Model file for the job. Use its own axes, mm. A direction names the side the tool comes from. Round coordinates to 2 decimals unless told otherwise and drop trailing zeros. Order: outer loops, then holes, each group sorted by start corner. A loop starts at its lowest first (then second) coordinate and runs counter-clockwise, first axis right, second up. Notation, with made-up numbers: (-12, -6) -> (41, -6) arc R26 cw to (41, 16) -> close; hole circle Ø6 at (-31.5, 8). An arc over 180 degrees is marked (long way). Put each result on its own line as item: value. Start each with the question number.
Q1. Pull direction Y, two halves, no side cores. Call faces 4 (the face through (-1.46, -6.59, 40.6)), 5 (the face through (7.62, -3.16, 41.34)), 6 (the face through (-5.75, -5.27, 0.79)), 7 (the face through (-7, 0, 65)): released by +Y, released by -Y, zero draft, split by the parting line, or undercut.
Q2. Cut at A-A, the plane y = 0. List the corners of the cut face in (x, z).
Q3. Cut at D-D, the plane z = 11. List the corners of the cut face in (x, y).
Q4. Cut at C-C, the plane z = 58.5. List the corners of the cut face in (x, y), and give its area (3 significant figures).
Q5. Probe L1, parallel to Y at x = 0, z = 0.85; L2, parallel to Z at x = -6.25, y = 3.75; L3, parallel to Y at x = 0.25, z = 16.5. List the from-to ranges inside material, lowest first.
Q6. Flat gauge pins, fed straight in: P1, Ø6, axis at x = 1.5, z = 41.5, coming from the +Y side; P2, Ø2, axis at x = 4.5, z = 50, coming from the +Y side; P3, Ø4, axis at y = 4, z = 52, coming from the -X side. Where does each tip first touch, or does it go through?
Q7. 3-axis set-ups, long thin cutter, end or side, ignore diameter. For faces 1 (the face through (0, 0, 1.6)), 2 (the face through (-1.73, -7.81, 9.21)), 3 (the face through (-3, 8, 17)): which of +Z, -Z, +X, -X, +Y, -Y reach the whole face in a straight line?
from build123d import *

# Parameters (mm, degrees)
F0_R     = 9.5
F1_DEPTH = 65
F2_R     = 0.2
F3_R     = 9.5
F3_R_2   = 8.25
F4_DEPTH = 48
F5_R     = 7.8
F6_DEPTH = 1.6
F7_T     = -1.5


with BuildPart() as f1:
    # F0 (on Top) → F1 (new body)
    with BuildSketch(Plane.XY):
        Circle(F0_R)
    extrude(amount=F1_DEPTH)

    # F2
    f2_edges = [f1.edges().sort_by_distance(p)[0] for p in [
        (-9.5, 0, 0),
    ]]
    fillet(f2_edges, radius=F2_R)

    # F3 (on face) → F4 (cut)
    with BuildSketch(Plane.XY.offset(65)):
        Circle(F3_R)
        Circle(F3_R_2, mode=Mode.SUBTRACT)
    extrude(amount=-F4_DEPTH, mode=Mode.SUBTRACT)

    # F5 (on face) → F6 (cut)
    with BuildSketch(Plane(origin=(0, 0, 0), x_dir=(1, 0, 0), z_dir=(0, 0, -1))):
        Circle(F5_R)
    extrude(amount=-F6_DEPTH, mode=Mode.SUBTRACT)

    # F7
    f7_openings = [f1.faces().sort_by_distance(p)[0] for p in [
        (0, 0, 65),
    ]]
    offset(amount=F7_T, openings=f7_openings, kind=Kind.INTERSECTION)


solid = f1.part
Ans:
1. face 4: undercut
1. face 5: split by the parting line
1. face 6: undercut
1. face 7: zero draft
2. outline: (-9.5, 0.2) arc R0.2 ccw to (-9.3, 0) -> (-7.8, 0) -> (-7.8, 1.6) -> (7.8, 1.6) -> (7.8, 0) -> (9.3, 0) arc R0.2 ccw to (9.5, 0.2) -> (9.5, 17) -> (8.25, 17) -> (8.25, 65) -> (6.75, 65) -> (6.75, 15.5) -> (8, 15.5) -> (8, 3.1) -> (-8, 3.1) -> (-8, 15.5) -> (-6.75, 15.5) -> (-6.75, 65) -> (-8.25, 65) -> (-8.25, 17) -> (-9.5, 17) -> close
3. outline: circle Ø19 at (0, 0); hole circle Ø16 at (0, 0)
4. outline: circle Ø16.5 at (0, 0); hole circle Ø13.5 at (0, 0)
4. area: 70.7 mm^2
5. L1: y = -9.5 to -7.8, 7.8 to 9.5
5. L2: z = 1.6 to 3.1, 15.5 to 65
5. L3: y = -9.5 to -6.75, 6.75 to 9.5
6. P1: stops at y = 8.25
6. P2: stops at y = 7.47
6. P3: stops at x = -8
7. face 1: -Z
7. face 2: none
7. face 3: +Z
